from build123d import *

# Parameters (mm, degrees)
SKETCH1_R           = 3.4
BOSS_EXTRUDE2_DEPTH = 100
FILLET5_R           = 2.5
FILLET6_R           = 1.5
FILLET7_R           = 1.5
FILLET8_R           = 1
SKETCH3_R           = 3.4
BOSS_EXTRUDE4_DEPTH = 200


with BuildPart() as part:
    # Sketch1 → Boss-Extrude2 (new body)
    with BuildSketch(Plane(origin=(0, 0, 0), x_dir=(0, 0, -1), z_dir=(1, 0, 0))):
        Polygon((10.9, 0), (10.9, 2.4), (6.75, 2.4), (6.75, 5.05), (10.9, 9.2), (19.1, 9.2), (23.25, 5.05), (23.25, 2.4), (19.1, 2.4), (19.1, 0), (30, 0), (30, 10.9), (27.6, 10.9), (27.6, 6.75), (24.95, 6.75), (20.8, 10.9), (20.8, 19.1), (24.95, 23.25), (27.6, 23.25), (27.6, 19.1), (30, 19.1), (30, 30), (19.1, 30), (19.1, 27.6), (23.25, 27.6), (23.25, 24.95), (19.1, 20.8), (10.9, 20.8), (6.75, 24.95), (6.75, 27.6), (10.9, 27.6), (10.9, 30), (0, 30), (0, 19.1), (2.4, 19.1), (2.4, 23.25), (5.05, 23.25), (9.2, 19.1), (9.2, 10.9), (5.05, 6.75), (2.4, 6.75), (2.4, 10.9), (0, 10.9), (0, 0), align=None)
        with Locations((15, 15)):
            Circle(SKETCH1_R, mode=Mode.SUBTRACT)
    extrude(amount=BOSS_EXTRUDE2_DEPTH)

    # Fillet5
    fillet5_edges = [part.edges().sort_by_distance(p)[0] for p in [
        (50, 30, 0),
        (50, 30, -30),
        (50, 0, -30),
        (50, 0, 0),
    ]]
    fillet(fillet5_edges, radius=FILLET5_R)

    # Fillet6
    fillet6_edges = [part.edges().sort_by_distance(p)[0] for p in [
        (50, 10.9, -9.2),
        (50, 19.1, -9.2),
        (50, 19.1, -20.8),
        (50, 10.9, -20.8),
        (50, 9.2, -19.1),
        (50, 9.2, -10.9),
    ]]
    fillet(fillet6_edges, radius=FILLET6_R)

    # Fillet7
    fillet7_edges = [part.edges().sort_by_distance(p)[0] for p in [
        (50, 20.8, -10.9),
        (50, 20.8, -19.1),
    ]]
    fillet(fillet7_edges, radius=FILLET7_R)

    # Fillet8
    fillet8_edges = [part.edges().sort_by_distance(p)[0] for p in [
        (50, 6.75, -2.4),
        (50, 23.25, -2.4),
        (50, 27.6, -6.75),
        (50, 27.6, -23.25),
        (50, 23.25, -27.6),
        (50, 6.75, -27.6),
        (50, 2.4, -23.25),
        (50, 2.4, -6.75),
    ]]
    fillet(fillet8_edges, radius=FILLET8_R)

    # Sketch3 → Boss-Extrude4 (add)
    with BuildSketch(Plane(origin=(0, 0, 0), x_dir=(0, 0, -1), z_dir=(1, 0, 0))):
        with BuildLine():
            Line((10.9, 27.6), (10.9, 30))
            Line((10.9, 30), (2.5, 30))
            ThreePointArc((2.5, 30), (0.732233047, 29.267766953), (0, 27.5))
            Line((0, 27.5), (0, 19.1))
            Line((0, 19.1), (2.4, 19.1))
            Line((2.4, 19.1), (2.4, 22.25))
            ThreePointArc((2.4, 22.25), (2.692893219, 22.957106781), (3.4, 23.25))
            Line((3.4, 23.25), (5.05, 23.25))
            Line((5.05, 23.25), (8.760660172, 19.539339828))
            ThreePointArc((8.760660172, 19.539339828), (9.085819299, 19.052704805), (9.2, 18.478679656))
            Line((9.2, 18.478679656), (9.2, 11.521320344))
            ThreePointArc((9.2, 11.521320344), (9.085819299, 10.947295195), (8.760660172, 10.460660172))
            Line((8.760660172, 10.460660172), (5.05, 6.75))
            Line((5.05, 6.75), (3.4, 6.75))
            ThreePointArc((3.4, 6.75), (2.692893219, 7.042893219), (2.4, 7.75))
            Line((2.4, 7.75), (2.4, 10.9))
            Line((2.4, 10.9), (0, 10.9))
            Line((0, 10.9), (0, 2.5))
            ThreePointArc((0, 2.5), (0.732233047, 0.732233047), (2.5, 0))
            Line((2.5, 0), (10.9, 0))
            Line((10.9, 0), (10.9, 2.4))
            Line((10.9, 2.4), (7.75, 2.4))
            ThreePointArc((7.75, 2.4), (7.042893219, 2.692893219), (6.75, 3.4))
            Line((6.75, 3.4), (6.75, 5.05))
            Line((6.75, 5.05), (10.460660172, 8.760660172))
            ThreePointArc((10.460660172, 8.760660172), (10.947295195, 9.085819299), (11.521320344, 9.2))
            Line((11.521320344, 9.2), (18.478679656, 9.2))
            ThreePointArc((18.478679656, 9.2), (19.052704805, 9.085819299), (19.539339828, 8.760660172))
            Line((19.539339828, 8.760660172), (23.25, 5.05))
            Line((23.25, 5.05), (23.25, 3.4))
            ThreePointArc((23.25, 3.4), (22.957106781, 2.692893219), (22.25, 2.4))
            Line((22.25, 2.4), (19.1, 2.4))
            Line((19.1, 2.4), (19.1, 0))
            Line((19.1, 0), (27.5, 0))
            ThreePointArc((27.5, 0), (29.267766953, 0.732233047), (30, 2.5))
            Line((30, 2.5), (30, 10.9))
            Line((30, 10.9), (27.6, 10.9))
            Line((27.6, 10.9), (27.6, 7.75))
            ThreePointArc((27.6, 7.75), (27.307106781, 7.042893219), (26.6, 6.75))
            Line((26.6, 6.75), (24.95, 6.75))
            Line((24.95, 6.75), (21.239339828, 10.460660172))
            ThreePointArc((21.239339828, 10.460660172), (20.914180701, 10.947295195), (20.8, 11.521320344))
            Line((20.8, 11.521320344), (20.8, 18.478679656))
            ThreePointArc((20.8, 18.478679656), (20.914180701, 19.052704805), (21.239339828, 19.539339828))
            Line((21.239339828, 19.539339828), (24.95, 23.25))
            Line((24.95, 23.25), (26.6, 23.25))
            ThreePointArc((26.6, 23.25), (27.307106781, 22.957106781), (27.6, 22.25))
            Line((27.6, 22.25), (27.6, 19.1))
            Line((27.6, 19.1), (30, 19.1))
            Line((30, 19.1), (30, 27.5))
            ThreePointArc((30, 27.5), (29.267766953, 29.267766953), (27.5, 30))
            Line((27.5, 30), (19.1, 30))
            Line((19.1, 30), (19.1, 27.6))
            Line((19.1, 27.6), (22.25, 27.6))
            ThreePointArc((22.25, 27.6), (22.957106781, 27.307106781), (23.25, 26.6))
            Line((23.25, 26.6), (23.25, 24.95))
            Line((23.25, 24.95), (19.539339828, 21.239339828))
            ThreePointArc((19.539339828, 21.239339828), (19.052704805, 20.914180701), (18.478679656, 20.8))
            Line((18.478679656, 20.8), (11.521320344, 20.8))
            ThreePointArc((11.521320344, 20.8), (10.947295195, 20.914180701), (10.460660172, 21.239339828))
            Line((10.460660172, 21.239339828), (6.75, 24.95))
            Line((6.75, 24.95), (6.75, 26.6))
            ThreePointArc((6.75, 26.6), (7.042893219, 27.307106781), (7.75, 27.6))
            Line((7.75, 27.6), (10.9, 27.6))
        make_face()
        with Locations((15, 15)):
            Circle(SKETCH3_R, mode=Mode.SUBTRACT)
    extrude(amount=-BOSS_EXTRUDE4_DEPTH)


solid = part.part
Read the model definition and answer for the solid it produces. Units are mm, in the model's axes. A direction names the side the tool comes from. Round coordinates to 2 decimals unless told otherwise and drop trailing zeros. Write each loop counter-clockwise with the first axis right and the second up, starting at its lowest first coordinate (ties: lowest second). Pieces come first, ordered by that corner, then holes.
1. The part is cut by section B-B, the plane y = 15. Determine the outline of the cut face in (x, z), then the cut area to 3 significant figures.
2. The part is cut by section A-A, the plane z = -15. Determine the outline of the cut face in (x, y), then the cut area to 3 significant figures.
3. Determine the mould class of faces 6 (the face through (-48, 23, 0)), 7 (the face through (-48, 20.8, -15)), 8 (the face through (-52.1, 11.68, -14.26)), 9 (the face through (-48, 23, -30)) for opening direction Z: pulls with the +Z half, pulls with the -Z half, needs draft (parallel to the pull), parting line crosses it, or undercut.
4. Which of the six approach directions +Z, -Z, +X, -X, +Y, -Y give full straight-line access (tool end or side, diameter ignored) to faces 1 (the face through (-48, 15, -9.2)), 2 (the face through (-48, 30, -23)), 3 (the face through (-48, 0, -7)), 4 (the face through (-48, 15, -20.8)), 5 (the face through (-48, 9.2, -15))?
5. Given pin 1 Ø0.7 at (x, z) = (-116.5, -1.5) entering from -Y; pin 2 Ø5 at (x, y) = (-48, 16) entering from +Z; pin 3 Ø1 at (x, z) = (-11.5, -18) entering from +Y, each flat-ended and moving along its own axis, determine where each tip first touches the part or whether it passes through.
6. Straight lines are drawn through the part: L1, parallel to Z at x = -68.5, y = 20.5; L2, parallel to Y at x = -126, z = -9.5; L3, parallel to Z at x = -90, y = 10.5. For each, find the intervals that lie inside material, in ascending order.
Values:
1. outline: (-200, -20.8) - (100, -20.8) - (100, -18.4) - (-200, -18.4) - close; (-200, -11.6) - (100, -11.6) - (100, -9.2) - (-200, -9.2) - close
1. area: 1,440 mm2
2. outline: (-200, 9.2) - (100, 9.2) - (100, 11.6) - (-200, 11.6) - close; (-200, 18.4) - (100, 18.4) - (100, 20.8) - (-200, 20.8) - close
2. area: 1,440 mm2
3. face 6: pulls with the +Z half
3. face 7: undercut
3. face 8: undercut
3. face 9: pulls with the -Z half
4. face 1: +Z, +X, -X
4. face 2: +Z, -Z, +X, -X, +Y
4. face 3: +Z, -Z, +X, -X, -Y
4. face 4: -Z, +X, -X
4. face 5: +X, -X, -Y
5. pin 1: stops at y = 0.09
5. pin 2: stops at z = -9.2
5. pin 3: stops at y = 20.8
6. L1: z = -30 to -27.6, -22.2 to -7.8, -2.4 to 0
6. L2: y = 0 to 2.4, 7.8 to 22.2, 27.6 to 30
6. L3: z = -30 to -27.6, -21.2 to -8.8, -2.4 to 0
